```python
from build123d import *

# Parameters (mm, degrees)
SKETCH_1_R          = 11
EXTRUDE_1_DEPTH     = 3.5
SKETCH_2_R          = 4
CUT_EXTRUDE_1_DEPTH = 16.945218719
EXTRUDE_START       = 10
SKETCH_3_R          = 5.1
SKETCH_3_R_2        = 4
EXTRUDE_2_DEPTH     = 10
SKETCH_6_R          = 5.1
SKETCH_6_R_2        = 4
EXTRUDE_3_DEPTH     = 1.5
SKETCH_7_R          = 1.75
CUT_EXTRUDE_2_DEPTH = 19.493242009
CHAMFER_1_SIZE      = 0.5


with BuildPart() as part:
    # 草图1 → 凸台-拉伸1 (new body)
    with BuildSketch(Plane(origin=(0, 0, 0), x_dir=(1, 0, 0), z_dir=(0, 1, 0))):
        with Locations(Location((0, 0, 0), (0, 0, 270))):
            Circle(SKETCH_1_R)
    extrude(amount=EXTRUDE_1_DEPTH)

    # 草图2 → 切除-拉伸1 (cut, through all)
    with BuildSketch(Plane(origin=(0, 3.5, 0), x_dir=(1, 0, 0), z_dir=(0, 1, 0))):
        with Locations(Location((0, 0, 0), (0, 0, 270))):
            Circle(SKETCH_2_R)
    extrude(amount=-CUT_EXTRUDE_1_DEPTH, mode=Mode.SUBTRACT)

    # 草图3 → 凸台-拉伸2 (add)
    with BuildSketch(Plane(origin=(0, 3.5, 0), x_dir=(1, 0, 0), z_dir=(0, 1, 0)).offset(EXTRUDE_START)):
        with Locations(Location((0, 0, 0), (0, 0, 270))):
            Circle(SKETCH_3_R)
        with Locations(Location((0, 0, 0), (0, 0, 270))):
            Circle(SKETCH_3_R_2, mode=Mode.SUBTRACT)
    extrude(amount=-EXTRUDE_2_DEPTH)

    # 草图6 → 凸台-拉伸3 (add)
    with BuildSketch(Plane.XZ):
        with Locations(Location((0, 0, 0), (0, 0, 90))):
            Circle(SKETCH_6_R)
        with Locations(Location((0, 0, 0), (0, 0, 90))):
            Circle(SKETCH_6_R_2, mode=Mode.SUBTRACT)
    extrude(amount=EXTRUDE_3_DEPTH)

    # 草图7 → 切除-拉伸2 (cut, through all)
    with BuildSketch(Plane(origin=(0, 3.5, 0), x_dir=(1, 0, 0), z_dir=(0, 1, 0))):
        with Locations(Location((0, 8, 0), (0, 0, 270))):
            Circle(SKETCH_7_R)
        with Locations(Location((8, 0, 0), (0, 0, 270))):
            Circle(SKETCH_7_R)
        with Locations(Location((0, -8, 0), (0, 0, 270))):
            Circle(SKETCH_7_R)
        with Locations(Location((-8, 0, 0), (0, 0, 270))):
            Circle(SKETCH_7_R)
    extrude(amount=-CUT_EXTRUDE_2_DEPTH, mode=Mode.SUBTRACT)

    # 倒角1
    chamfer_1_edges = [part.edges().sort_by_distance(p)[0] for p in [
        (0, 13.5, -5.1),
        (0, -1.5, -5.1),
    ]]
    chamfer(chamfer_1_edges, length=CHAMFER_1_SIZE)


solid = part.part
```
The listing builds one solid part. Answer for the finished solid, in the listing's coordinates (mm). A direction names the side the tool comes from. Give positions to 0.01 mm unless a question says otherwise; leave off trailing zeros. Write each loop counter-clockwise with the first axis right and the second up, starting at its lowest first coordinate (ties: lowest second). Pieces come first, ordered by that corner, then holes. Notation, with made-up numbers: (5, 10.25) -> (51, 10.25) arc R5 cw to (51, 17.25) -> close; hole circle Ø6 at (8, -25.75). An arc over 180 degrees is marked (long way). Write item = value, one per line. Start each with the question number.
1) Straight lines are drawn through the part: line 1 along X through (y, z) = (1.2, 0); line 2 along Z through (x, y) = (0.75, 2); line 3 along X through (y, z) = (10.75, -2). For each, find the intervals that lie inside material, in ascending order.
2) The part is cut by section D-D, the plane z = 8. Determine the outline of the cut face in (x, y).
3) Determine the mould class of faces 1 (the face through (-2, 3.5, 5)), 2 (the face through (-0.67, 1.774, -6.383)), 3 (the face through (1.532, 8.317, 4.864)), 4 (the face through (0.526, 1.774, 9.669)) for opening direction X: +X half, -X half, draft (parallel to the pull), parting line (faces both ways), or undercut.
4) Which of the six approach directions +Z, -Z, +X, -X, +Y, -Y give full straight-line access (tool end or side, diameter ignored) to faces 5 (the face through (-2, 0, 5)), 6 (the face through (-3.8, -1.5, -1.7))?
5) The part is cut by section C-C, the plane x = -6.75. Determine the outline of the cut face in (y, z).
6) The part is cut by section A-A, the plane x = 0. Determine the outline of the cut face in (y, z), and give its area (3 significant figures).
7) Each of these flat-tipped pins is pushed along its axis until it touches: pin 1 (4 mm diameter, centred on y = 10.5, z = 2, fed in from +X); pin 2 (6.5 mm diameter, centred on x = 3.5, z = 4.5, fed in from +Y); pin 3 (4 mm diameter, centred on x = 0, z = -8, fed in from +Y); pin 4 (2 mm diameter, centred on x = -2.5, y = 1, fed in from +Z). Where does it stop, or does it pass through?
8) The part is cut by section B-B, the plane z = 0. Determine the outline of the cut face in (x, y), and give its area (3 significant figures).
Solutions:
q1.line_1 = -11 to -9.75, -6.25 to -4, 4 to 6.25, 9.75 to 11
q1.line_2 = -10.97 to -9.58, -6.42 to -3.93, 3.93 to 6.42, 9.58 to 10.97
q1.line_3 = -4.69 to -3.46, 3.46 to 4.69
q2.outline = (-7.55, 0) -> (-1.75, 0) -> (-1.75, 3.5) -> (-7.55, 3.5) -> close; (1.75, 0) -> (7.55, 0) -> (7.55, 3.5) -> (1.75, 3.5) -> close
q3.face_1 = draft
q3.face_2 = undercut
q3.face_3 = parting line
q3.face_4 = undercut
q4.face_5 = -Y
q4.face_6 = +Z, -Z, +X, -X, -Y
q5.outline = (0, -8.69) -> (3.5, -8.69) -> (3.5, -1.22) -> (0, -1.22) -> close; (0, 1.22) -> (3.5, 1.22) -> (3.5, 8.69) -> (0, 8.69) -> close
q6.outline = (-1.5, -4.6) -> (-1, -5.1) -> (0, -5.1) -> (0, -6.25) -> (3.5, -6.25) -> (3.5, -5.1) -> (13, -5.1) -> (13.5, -4.6) -> (13.5, -4) -> (-1.5, -4) -> close; (-1.5, 4) -> (13.5, 4) -> (13.5, 4.6) -> (13, 5.1) -> (3.5, 5.1) -> (3.5, 6.25) -> (0, 6.25) -> (0, 5.1) -> (-1, 5.1) -> (-1.5, 4.6) -> close; (0, -11) -> (3.5, -11) -> (3.5, -9.75) -> (0, -9.75) -> close; (0, 9.75) -> (3.5, 9.75) -> (3.5, 11) -> (0, 11) -> close
q6.area = 49.3 mm²
q7.pin_1 = 5.1
q7.pin_2 = 13.5
q7.pin_3 = 3.5
q7.pin_4 = 10.9
q8.outline = (-11, 0) -> (-9.75, 0) -> (-9.75, 3.5) -> (-11, 3.5) -> close; (-6.25, 0) -> (-5.1, 0) -> (-5.1, -1) -> (-4.6, -1.5) -> (-4, -1.5) -> (-4, 13.5) -> (-4.6, 13.5) -> (-5.1, 13) -> (-5.1, 3.5) -> (-6.25, 3.5) -> close; (4, -1.5) -> (4.6, -1.5) -> (5.1, -1) -> (5.1, 0) -> (6.25, 0) -> (6.25, 3.5) -> (5.1, 3.5) -> (5.1, 13) -> (4.6, 13.5) -> (4, 13.5) -> close; (9.75, 0) -> (11, 0) -> (11, 3.5) -> (9.75, 3.5) -> close
q8.area = 49.3 mm²
